Read the model definition and answer for the solid it produces. Units are mm, in the model's axes. A direction names the side the tool comes from. Coordinates: 2 decimals unless noted, no trailing zeros. Loops run counter-clockwise (first coordinate to the right, second up) from the corner with the lowest first, then second, coordinate; pieces in that order, holes last.
from build123d import *

# Parameters (mm, degrees)
SKETCH_R     = 16.5
SKETCH_R_2   = 3
SKETCH_R_3   = 4.2
PAD_DEPTH    = 2
SKETCH001_W  = 2
SKETCH001_H  = 2
POCKET_DEPTH = 2.001


with BuildPart() as part:
    # Sketch → Pad (new body)
    with BuildSketch(Plane.XY):
        Circle(SKETCH_R)
        with Locations((-11.5, 0)):
            Circle(SKETCH_R_2, mode=Mode.SUBTRACT)
        with Locations((11.5, 0)):
            Circle(SKETCH_R_2, mode=Mode.SUBTRACT)
        Circle(SKETCH_R_3, mode=Mode.SUBTRACT)
    extrude(amount=PAD_DEPTH)

    # Sketch001 → Pocket (cut, through all)
    with BuildSketch(Plane.XY.offset(2)):
        with Locations((0, 4)):
            Rectangle(SKETCH001_W, SKETCH001_H)
    extrude(amount=-POCKET_DEPTH, mode=Mode.SUBTRACT)


solid = part.part
Item 1: Determine the mould class of faces 3 (the face through (3.4, -3.4, 2)), 4 (the face through (15.24, -6.32, 0.99)), 5 (the face through (-13.9, -1.8, 1)) for opening direction Y: released by +Y, released by -Y, zero draft, split by the parting line, or undercut.
Numbers:
face 3: zero draft
face 4: split by the parting line
face 5: undercut
Item 2: A cutting plane is placed at D-D on y = -6.5. Determine the outline of the cut face in (x, z).
Numbers:
outline: (-15.17, 0) - (15.17, 0) - (15.17, 2) - (-15.17, 2) - close
Item 3: A cutting plane is placed at C-C on x = -11.5. Determine the outline of the cut face in (y, z), then the cut area to 3 significant figures.
Numbers:
outline: (-11.83, 0) - (-3, 0) - (-3, 2) - (-11.83, 2) - close; (3, 0) - (11.83, 0) - (11.83, 2) - (3, 2) - close
area: 35.3 mm2
Item 4: A cutting plane is placed at A-A on x = 0. Determine the outline of the cut face in (y, z), then the cut area to 3 significant figures.
Numbers:
outline: (-16.5, 0) - (-4.2, 0) - (-4.2, 2) - (-16.5, 2) - close; (5, 0) - (16.5, 0) - (16.5, 2) - (5, 2) - close
area: 47.6 mm2
Item 5: Which of the six approach directions +Z, -Z, +X, -X, +Y, -Y give full straight-line access (tool end or side, diameter ignored) to faces 1 (the face through (1, 4.5, 1)), 2 (the face through (3.4, -3.4, 0))?
Numbers:
face 1: +Z, -Z
face 2: -Z, +X, -X, +Y, -Y
Item 6: A cutting plane is placed at B-B on y = 0. Determine the outline of the cut face in (x, z).
Numbers:
outline: (-16.5, 0) - (-14.5, 0) - (-14.5, 2) - (-16.5, 2) - close; (-8.5, 0) - (-4.2, 0) - (-4.2, 2) - (-8.5, 2) - close; (4.2, 0) - (8.5, 0) - (8.5, 2) - (4.2, 2) - close; (14.5, 0) - (16.5, 0) - (16.5, 2) - (14.5, 2) - close
Item 7: Find the intervals of material crossed by line 1 along Y through (x, z) = (0, 0.7); line 2 along X through (y, z) = (1.5, 1.7); line 3 along X through (y, z) = (-2, 0.65), in increasing order.
Numbers:
line 1: y = -16.5 to -4.2, 5 to 16.5
line 2: x = -16.43 to -14.1, -8.9 to -3.92, 3.92 to 8.9, 14.1 to 16.43
line 3: x = -16.38 to -13.74, -9.26 to -3.69, 3.69 to 9.26, 13.74 to 16.38
Item 8: Given pin 1 (13.5 mm diameter, centred on x = 0, y = 0, fed in from -Z); pin 2 (1 mm diameter, centred on y = 4.5, z = 0.5, fed in from -X); pin 3 (0.7 mm diameter, centred on y = 4.5, z = 0.5, fed in from +X), each flat-ended and moving along its own axis, determine where each tip first touches the part or whether it passes through.
Numbers:
pin 1: stops at z = 0
pin 2: stops at x = -16.01
pin 3: stops at x = 15.97
